from build123d import *

# Parameters (mm, degrees)
SKETCH1_R           = 1.7
BOSS_EXTRUDE1_DEPTH = 30
SKETCH2_W           = 13
SKETCH2_H           = 24
SKETCH2_W_2         = 7.133537961
CUT_EXTRUDE2_DEPTH  = 30
SKETCH3_W           = 16.393620584
SKETCH3_H           = 16
CUT_EXTRUDE3_DEPTH  = 30
CUT_EXTRUDE4_DEPTH  = 3.5
CUT_EXTRUDE5_DEPTH  = 78.230456788


with BuildPart() as part:
    # Sketch1 → Boss-Extrude1 (new body)
    with BuildSketch(Plane(origin=(0, 0, 0), x_dir=(1, 0, 0), z_dir=(0, 1, 0))):
        with BuildLine():
            Line((0.547347337, 46.773363131), (-12.096275709, 67.916751063))
            ThreePointArc((-12.096275709, 67.916751063), (-15.207212104, 69.964878097), (-18.746235825, 68.803817933))
            Line((-18.746235825, 68.803817933), (-21.570135396, 67.115142409))
            Line((-21.570135396, 67.115142409), (-6.784148434, 42.389171288))
            ThreePointArc((-6.784148434, 42.389171288), (-0.926304627, 40.915519323), (0.547347337, 46.773363131))
        make_face()
        with Locations(Location((-3.118400548, 44.581267209, 0), (0, 0, 270))):
            Circle(SKETCH1_R, mode=Mode.SUBTRACT)
        with Locations(Location((-15.773770801, 65.71763038, 0), (0, 0, 270))):
            Circle(SKETCH1_R, mode=Mode.SUBTRACT)
    extrude(amount=BOSS_EXTRUDE1_DEPTH)

    # Sketch2 → Cut-Extrude2 (cut)
    with BuildSketch(Plane(origin=(13.674403301, 0, -8.177213665), x_dir=(0.5132293910361586, 0, 0.8582514737398672), z_dir=(-0.8582514737398672, 0, 0.5132293910361586))):
        with Locations((-62.172097336, 15)):
            Rectangle(SKETCH2_W, SKETCH2_H)
        with Locations((-72.238866317, 15)):
            Rectangle(SKETCH2_W_2, SKETCH2_H)
    extrude(amount=-CUT_EXTRUDE2_DEPTH, mode=Mode.SUBTRACT)

    # Sketch3 → Cut-Extrude3 (cut)
    with BuildSketch(Plane(origin=(13.674403301, 0, -8.177213665), x_dir=(0.5132293910361586, 0, 0.8582514737398672), z_dir=(-0.8582514737398672, 0, 0.5132293910361586))):
        with Locations((-37.475287044, 15)):
            Rectangle(SKETCH3_W, SKETCH3_H)
    extrude(amount=-CUT_EXTRUDE3_DEPTH, mode=Mode.SUBTRACT)

    # Sketch7 → Cut-Extrude4 (cut)
    with BuildSketch(Plane(origin=(0, 0, 0), x_dir=(-1, 0, 0), z_dir=(0, -1, 0))):
        Polygon((1.817751365, 50.728416138), (9.149247136, 46.344224296), (4.210618406, 38.085567524), (-3.391020631, 42.018010382), align=None)
    extrude(amount=-CUT_EXTRUDE4_DEPTH, mode=Mode.SUBTRACT)

    # Sketch9 → Cut-Extrude5 (cut, through all)
    with BuildSketch(Plane(origin=(13.674403301, 0, -8.177213665), x_dir=(0.5132293910361586, 0, 0.8582514737398672), z_dir=(-0.8582514737398672, 0, 0.5132293910361586))):
        Polygon((-44.470661337, 30), (-44.470661337, 26.5), (-33.41668301, 26.5), (-33.41668301, 30.544862053), (-44.470661337, 30.544862053), align=None)
    extrude(amount=-CUT_EXTRUDE5_DEPTH, mode=Mode.SUBTRACT)


solid = part.part
Geometry: final body of the model. Coordinates: model frame, mm. A direction names the side the tool comes from. Give positions to 0.01 mm unless a question says otherwise; leave off trailing zeros. Loops run counter-clockwise (first coordinate to the right, second up) from the corner with the lowest first, then second, coordinate; pieces in that order, holes last. Notation, with made-up numbers: (22, -13) -> (55, -13) arc R22 cw to (55, 14) -> close; hole circle Ø9 at (48.5, 14.25). An arc over 180 degrees is marked (long way). Put each result on its own line as item: value.
1. Ray query, line 1 along Y through (x, z) = (-0.75, -42.5); line 2 along Z through (x, y) = (-9.25, 22); line 3 along X through (y, z) = (26, -49). Return the intervals inside material, ascending. Write a range as [from, to].
Taken from the geometry:
line 1: y = [3.5, 7], [23, 26.5]
line 2: z = [-59.34, -47.68]
line 3: x = [-10.74, -0.78]
2. Pin query (flat end, axial travel): P1, Ø8, axis at y = 15.5, z = -45.5, coming from the -X side; P2, Ø1.5, axis at y = 4.5, z = -46.5, coming from the -X side; P3, Ø3, axis at x = -15.77, z = -65.72, coming from the +Y side; P4, Ø8, axis at y = 17, z = -55, coming from the -X side. Return the tip coordinate at first contact, or that it passes through.
Taken from the geometry:
P1: stops at x = -11.04
P2: stops at x = -9.69
P3: passes through
P4: stops at x = -14.9
3. Pull-direction query (Z, two-part tool) for faces 1 (the flat face through (-11.28, 14.83, -58.12)), 2 (the cylindrical face through (-2.61, 5.23, -42.96)), 3 (the flat face through (-4, 3.5, -47)), 4 (the flat face through (-6.151, 14.888, -49.537)); classes: released by +Z, released by -Z, zero draft, split by the parting line, or undercut.
Taken from the geometry:
face 1: released by -Z
face 2: undercut
face 3: zero draft
face 4: released by +Z
4. Cut plane B-B (x = -4). Return the cut outline in (y, z).
Taken from the geometry:
outline: (0, -54.38) -> (30, -54.38) -> (30, -49.42) -> (26.5, -49.42) -> (26.5, -46.03) -> (23, -46.03) -> (23, -50.82) -> (7, -50.82) -> (7, -46.03) -> (3.5, -46.03) -> (3.5, -49.42) -> (0, -49.42) -> close; (3.5, -43.13) -> (7, -43.13) -> (7, -40.4) -> (3.5, -40.4) -> close; (23, -43.13) -> (26.5, -43.13) -> (26.5, -40.4) -> (23, -40.4) -> close
5. Cut plane C-C (x = -18.25). Return the cut outline in (y, z), plus the area to 3 significant figures.
Taken from the geometry:
outline: (0, -69.21) -> (3, -69.21) -> (3, -61.56) -> (0, -61.56) -> close; (27, -69.21) -> (30, -69.21) -> (30, -61.56) -> (27, -61.56) -> close
area: 45.9 mm2
6. Set-up query: faces 5 (the flat face through (-4.3, 26.5, -46.4)), 6 (the flat face through (-4.2, 7, -46.2)), 7 (the flat face through (-15, 27, -64)). Return all of +Z, -Z, +X, -X, +Y, -Y with unobstructed straight access to the full face (end or side cutting, diameter ignored); none if empty.
Taken from the geometry:
face 5: +Z, +X, +Y
face 6: +Z, +X
face 7: -Z, -X
7. Cut plane A-A (z = -65.5). Return the cut outline in (x, y), plus the area to 3 significant figures.
Taken from the geometry:
outline: (-20.6, 0) -> (-17.46, 0) -> (-17.46, 3) -> (-20.6, 3) -> close; (-20.6, 27) -> (-17.46, 27) -> (-17.46, 30) -> (-20.6, 30) -> close; (-14.09, 0) -> (-10.65, 0) -> (-10.65, 3) -> (-14.09, 3) -> close; (-14.09, 27) -> (-10.65, 27) -> (-10.65, 30) -> (-14.09, 30) -> close
area: 39.5 mm2
8. Cut plane D-D (z = -62.25). Return the cut outline in (x, y).
Taken from the geometry:
outline: (-18.66, 0) -> (-8.71, 0) -> (-8.71, 3) -> (-18.66, 3) -> close; (-18.66, 27) -> (-8.71, 27) -> (-8.71, 30) -> (-18.66, 30) -> close
